from build123d import *

# Parameters (mm, degrees)
BASPROSKE_W     = 5
BASPROSKE_H     = 9
TOOTHCUT_DEPTH  = 14.674794331
TEETHCUTS_COUNT = 10
TEETHCUTS_ANGLE = 324
BORE_DEPTH      = 50.0003048


with BuildPart() as part:
    # BasProSke → Base-Revolve (revolve)
    with BuildSketch(Plane(origin=(0, 0, 0), x_dir=(1, 0, 0), z_dir=(0, 1, 0)), mode=Mode.PRIVATE) as base_revolve_sk:
        with Locations((2.5, 4.5)):
            Rectangle(BASPROSKE_W, BASPROSKE_H)
    revolve(base_revolve_sk.sketch.rotate(Axis((-10, 0, 0), (1, 0, 0)), 180), axis=Axis((-10, 0, 0), (1, 0, 0)))

    # TooCutSke → ToothCut (cut, through all)
    with BuildSketch(Plane(origin=(0, 0, 0), x_dir=(0, 0, -1), z_dir=(1, 0, 0))):
        with BuildLine():
            ThreePointArc((0.883878355, 5.554109745), (0, 5.624), (-0.883878355, 5.554109745))
            ThreePointArc((-0.883878355, 5.554109745), (-1.258245767, 7.379188248), (-2.637816971, 8.631324741))
            ThreePointArc((-2.637816971, 8.631324741), (0, 9.0254), (2.637816971, 8.631324741))
            ThreePointArc((2.637816971, 8.631324741), (1.258245767, 7.379188248), (0.883878355, 5.554109745))
        make_face()
    toothcut = extrude(amount=TOOTHCUT_DEPTH, mode=Mode.SUBTRACT)

    # TeethCuts: ToothCut ×10 about axis
    teethcuts_axis = Axis((-10, 0, 0), (1, 0, 0))
    for i in range(1, TEETHCUTS_COUNT):
        add(toothcut.rotate(teethcuts_axis, i * TEETHCUTS_ANGLE / (TEETHCUTS_COUNT - 1)), mode=Mode.SUBTRACT)

    # BorSke → Bore (cut, symmetric)
    with BuildSketch(Plane(origin=(0, 0, 0), x_dir=(0, 0, -1), z_dir=(1, 0, 0))):
        Polygon((0, 3.75), (-3.247595264, 1.875), (-3.247595264, -1.875), (0, -3.75), (3.247595264, -1.875), (3.247595264, 1.875), align=None)
    extrude(amount=BORE_DEPTH, both=True, mode=Mode.SUBTRACT)


solid = part.part
Model file for the job. Use its own axes, mm. Coordinates: 2 decimals unless noted, no trailing zeros. Order: outer loops, then holes, each group sorted by start corner. A loop starts at its lowest first (then second) coordinate and runs counter-clockwise, first axis right, second up. Notation, with made-up numbers: (74, 9) -> (120, 9) arc R23 cw to (120, 43) -> close; hole circle Ø7 at (-1.5, -39). An arc over 180 degrees is marked (long way). Return JSON: item names as keys, results as strings. Group by question number.
Item 1: Flat gauge pins, fed straight in: P1, Ø1.5, axis at x = 2.5, z = 6, coming from the -Y side; P2, Ø3, axis at x = 3, y = -5.5, coming from the +Z side; P3, Ø1.5, axis at x = 4, z = -0.5, coming from the +Y side. Where does each tip first touch, or does it go through?
Item 2: Saw through at A-A on y = 6.75. Write the cut outline in (x, z).
Item 3: Saw through at B-B on y = -7. Write the cut outline in (x, z).
Item 4: Wall check: line 1 along Z through (x, y) = (2.5, 5.25); line 2 along Y through (x, z) = (1.3, -6.75); line 3 along Z through (x, y) = (3.9, -4.5). Give the ranges that are in metal, low to high. Write a range as [from, to].
Values found:
{
 "1": {"P1": "stops at y = -5.5", "P2": "stops at z = 7.39", "P3": "stops at y = 7.36"},
 "2": {"outline": "(0, -3.32) -> (5, -3.32) -> (5, -0.99) -> (0, -0.99) -> close; (0, 0.99) -> (5, 0.99) -> (5, 3.32) -> (0, 3.32) -> close"},
 "3": {"outline": "(0, -3.34) -> (5, -3.34) -> (5, -1.08) -> (0, -1.08) -> close; (0, 1.08) -> (5, 1.08) -> (5, 3.34) -> (0, 3.34) -> close"},
 "4": {"line 1": "z = [-7.31, -5.4], [-2.75, 2.75], [5.4, 7.31]", "line 2": "y = [-5.49, -3.62], [-1.15, 1.15], [3.62, 5.49]", "line 3": "z = [-7.24, -4.36], [-3.37, 3.37], [4.36, 7.24]"}
}
